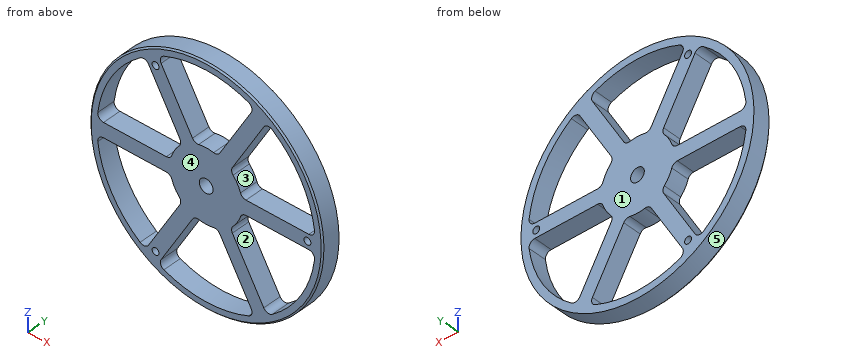
from build123d import *

# Parameters (mm, degrees)
F_12_0_189_DIAMETER_HOLE1_D  = 4.8006
CIRPATTERN3_COUNT            = 3
CUT_EXTRUDE1_DEPTH           = 115.6206569515286
FILLET1_R                    = 4
CIRPATTERN4_COUNT            = 6
FILLET1_OF_CIRPATTERN4_R     = 4
CHAMFER2_SIZE                = 1
F_3_8_0_375_DIAMETER_HOLE1_D = 9.525


with BuildPart() as part:
    # Sketch2 → Revolve1 (revolve)
    with BuildSketch(Plane(origin=(0, 0, 0), x_dir=(0, 0, -1), z_dir=(1, 0, 0)), mode=Mode.PRIVATE) as revolve1_sk:
        Polygon((0, 0), (-80.55, -9.86e-15), (-80.55, 12.699999999999989), (0, 12.699999999999989), align=None)
    revolve(revolve1_sk.sketch.rotate(Axis((0, -0.6350000000000106, 0), (0, 1, 0)), 180), axis=Axis((0, -0.6350000000000106, 0), (0, 1, 0)))

    # #12 (0.189) Diameter Hole1 (through all)
    with Locations(Plane(origin=(0, 12.699999999999989, 0), x_dir=(1, 0, 0), z_dir=(0, 1, 0))):
        with Locations((-35, 60.621778265)):
            f_12_0_189_diameter_hole1 = Hole(F_12_0_189_DIAMETER_HOLE1_D / 2)

    # CirPattern3: #12 (0.189) Diameter Hole1 ×3 about axis
    cirpattern3_axis = Axis((2.7e-16, 0, 4.47e-15), (0, 1, 0))
    for i in range(1, CIRPATTERN3_COUNT):
        add(f_12_0_189_diameter_hole1.rotate(cirpattern3_axis, i * 360 / CIRPATTERN3_COUNT), mode=Mode.SUBTRACT)

    # Sketch8 → Cut-Extrude1 (cut, through all)
    with BuildSketch(Plane(origin=(0, 12.699999999999989, 0), x_dir=(1, 0, 0), z_dir=(0, 1, 0))):
        with BuildLine():
            Line((-7.91732169499373, 23.713203435596423), (-33.36205552600357, 67.784775215972))
            ThreePointArc((-33.36205552600357, 67.784775215972), (4.63e-15, 75.54999999999998), (33.36205552600357, 67.784775215972))
            Line((33.36205552600357, 67.784775215972), (7.917321694993729, 23.713203435596423))
            ThreePointArc((7.917321694993729, 23.713203435596423), (1.53e-15, 25.000000000000007), (-7.91732169499373, 23.713203435596423))
        make_face()
    cut_extrude1 = extrude(amount=-CUT_EXTRUDE1_DEPTH, mode=Mode.SUBTRACT)

    # Fillet1
    fillet1_edges = [part.edges().sort_by_distance(p)[0] for p in [
        (7.9173216949937295, 6.349999999999994, -23.713203435596427),
        (-7.9173216949937295, 6.349999999999994, -23.713203435596427),
        (-33.36205552600357, 6.349999999999994, -67.78477521597199),
        (33.36205552600358, 6.349999999999994, -67.78477521597199),
    ]]
    fillet(fillet1_edges, radius=FILLET1_R)

    # CirPattern4: Cut-Extrude1 ×6 about axis
    cirpattern4_axis = Axis((-3.068e-14, 0, 1.3e-16), (0, 1, 0))
    for i in range(1, CIRPATTERN4_COUNT):
        add(cut_extrude1.rotate(cirpattern4_axis, i * 360 / CIRPATTERN4_COUNT), mode=Mode.SUBTRACT)

    # Fillet1 of CirPattern4
    fillet1_of_cirpattern4_edges = [part.edges().sort_by_distance(p)[0] for p in [
        (-16.57757573283808, 6.349999999999994, -18.71320343559648),
        (-24.494897427831813, 6.349999999999994, -5.000000000000001),
        (-75.38436508985136, 6.349999999999994, -4.999999999999924),
        (-42.02230956384777, 6.349999999999994, -62.78477521597215),
        (-24.49489742783184, 6.349999999999994, 4.99999999999994),
        (-16.577575732838117, 6.349999999999994, 18.713203435596423),
        (-42.02230956384782, 6.349999999999994, 62.78477521597206),
        (-75.38436508985139, 6.349999999999994, 4.999999999999838),
        (-7.9173216949937935, 6.349999999999994, 23.713203435596427),
        (7.917321694993666, 6.349999999999994, 23.713203435596427),
        (33.3620555260035, 6.349999999999994, 67.78477521597199),
        (-33.36205552600365, 6.349999999999994, 67.78477521597199),
        (16.57757573283801, 6.349999999999994, 18.71320343559649),
        (24.49489742783175, 6.349999999999994, 5.0000000000000115),
        (75.3843650898513, 6.349999999999994, 4.999999999999952),
        (42.022309563847685, 6.349999999999994, 62.78477521597216),
        (24.494897427831784, 6.349999999999994, -4.999999999999948),
        (16.577575732838053, 6.349999999999994, -18.71320343559643),
        (42.02230956384774, 6.349999999999994, -62.784775215972076),
        (75.38436508985133, 6.349999999999994, -4.999999999999863),
    ]]
    fillet(fillet1_of_cirpattern4_edges, radius=FILLET1_OF_CIRPATTERN4_R)

    # Chamfer2
    chamfer2_edges = [part.edges().sort_by_distance(p)[0] for p in [
        (-1.973e-14, -9.88e-15, 80.55),
    ]]
    chamfer(chamfer2_edges, length=CHAMFER2_SIZE)

    # 3/8 (0.375) Diameter Hole1 (through all)
    with Locations(Plane(origin=(0, 0, 0), x_dir=(-1, 0, 0), z_dir=(0, -1, 0))):
        with Locations((0, 0)):
            Hole(F_3_8_0_375_DIAMETER_HOLE1_D / 2)


solid = part.part
Verification items for the finished model (mm, model axes). Face numbers are marked on the shaded views. A direction names the side the tool comes from. Round coordinates to 2 decimals unless told otherwise and drop trailing zeros. Order: outer loops, then holes, each group sorted by start corner. A loop starts at its lowest first (then second) coordinate and runs counter-clockwise, first axis right, second up.
1. Thickness scan on L1, parallel to Z at x = 18.5, y = 8.25; L2, parallel to X at y = 8, z = 13; L3, parallel to X at y = 8.75, z = 54. Record the ranges inside material, lowest first.
Final values:
L1: z = -78.4 to -73.25, -42.04 to -22.04, -16.82 to 16.82, 22.04 to 42.04, 73.25 to 78.4
L2: x = -79.49 to -74.42, -21.35 to 21.35, 74.42 to 79.49
L3: x = -59.77 to -52.84, -36.95 to -25.4, 25.4 to 36.95, 52.84 to 59.77
2. Go/stop test with flat-tipped pins: P1, Ø5.5, axis at x = 70, z = 0, coming from the +Y side; P2, Ø8.5, axis at x = 0, z = 0, coming from the +Y side; P3, Ø1, axis at x = -5, y = 10, coming from the -Z side; P4, Ø1.5, axis at y = 9.5, z = 49.5, coming from the -X side. Record where each tip stops, or that it passes through.
Final values:
P1: stops at y = 12.7
P2: passes through
P3: stops at z = -80.42
P4: stops at x = -64.12
3. Section check C-C on y = 7. State how many separate pieces and enclosed holes the cut face has, then the cut area to 3 significant figures.
Final values:
separate pieces: 1
enclosed holes: 10
area: 7,400 mm2
4. Section check B-B on z = 0. Record the cut outline in (x, y), then the cut area to 3 significant figures.
Final values:
outline: (-80.55, 1) - (-79.55, 0) - (-4.76, 0) - (-4.76, 12.7) - (-80.55, 12.7) - close; (4.76, 0) - (67.6, 0) - (67.6, 12.7) - (4.76, 12.7) - close; (72.4, 0) - (79.55, 0) - (80.55, 1) - (80.55, 12.7) - (72.4, 12.7) - close
area: 1,860 mm2
5. Section check A-A on x = 0. Record the cut outline in (y, z).
Final values:
outline: (0, -79.55) - (1, -80.55) - (12.7, -80.55) - (12.7, -75.55) - (0, -75.55) - close; (0, -25) - (12.7, -25) - (12.7, -4.76) - (0, -4.76) - close; (0, 4.76) - (12.7, 4.76) - (12.7, 25) - (0, 25) - close; (0, 75.55) - (12.7, 75.55) - (12.7, 80.55) - (1, 80.55) - (0, 79.55) - close
6. Release check for a two-part mould opening along X. For the marked faces 3, 4 and 5 record: +X half, -X half, draft (parallel to the pull), parting line (faces both ways), or undercut.
Final values:
face 3: undercut
face 4: draft
face 5: parting line
7. Access from +Z, -Z, +X, -X, +Y, -Y to the whole of each face (thin tool, end or side, straight path). Record for the marked faces 1 and 2.
Final values:
face 1: +Z, -Z, +X, -X, +Y
face 2: +Y, -Y
